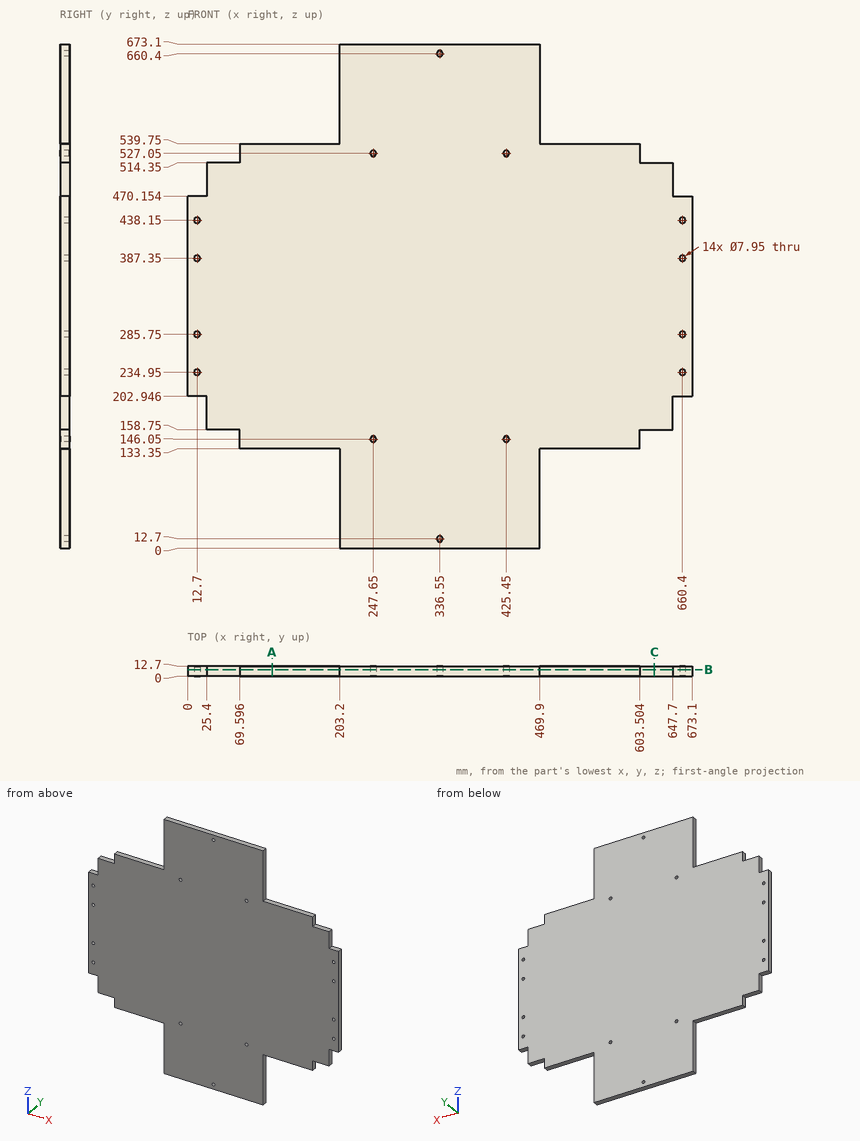
Geometry: see drawing. Coordinates: mm, zero at the bounding-box minimum. Coordinates: 2 decimals unless noted, no trailing zeros. Loops run counter-clockwise (first coordinate to the right, second up) from the corner with the lowest first, then second, coordinate; pieces in that order, holes last. Notation, with made-up numbers: M 24.5,-17.5 L 58.5,-17.5 A27 cw 58.5,12.5 Z; hole C 32.5,6.25 d1. An arc over 180 degrees is marked long. Put each result on its own line as item: value. Start each with the question number.
1) Contact query for flat-ended pins moving along their axis: pin 1 Ø5 at (y, z) = (11, 411) entering from -X; pin 2 Ø4 at (x, y) = (12.5, 8) entering from -Z; pin 3 Ø4 at (y, z) = (7.5, 141) entering from +X; pin 4 Ø6.5 at (y, z) = (4.5, 188) entering from +X. Output: stop coordinate, or through.
2) Cut plane A-A on x = 113. Return the cut outline in (y, z), then the cut area to 3 significant figures.
3) Cut plane C-C on x = 623. Return the cut outline in (y, z), then the cut area to 3 significant figures.
4) Ray query, L1, parallel to Z at x = 247.65, y = 7.75 (1 decimal); L2, parallel to X at y = 3.5, z = 438.15 (1 decimal). Return the intervals inside material, ascending. Write a range as from..to.
5) Cut plane B-B on y = 8.5. Give the number of separate pieces and of enclosed holes in the cut face, then the cut area to 3 significant figures.
The answers:
1. pin 1: stops at x = 0
1. pin 2: stops at z = 202.95
1. pin 3: stops at x = 603.5
1. pin 4: stops at x = 647.7
2. outline: M 0,133.35 L 12.7,133.35 L 12.7,539.75 L 0,539.75 Z
2. area: 5,160 mm²
3. outline: M 0,158.75 L 12.7,158.75 L 12.7,514.35 L 0,514.35 Z
3. area: 4,520 mm²
4. L1: z = 0..142.1, 150..523.1, 531..673.1
4. L2: x = 0..8.7, 16.7..656.4, 664.4..673.1
5. separate pieces: 1
5. enclosed holes: 14
5. area: 332,000 mm²
